Check sheet for the modelled part. Datum: model origin and axes. Units: mm. Face numbers are marked on the shaded views. Give positions to 0.01 mm unless a question says otherwise; leave off trailing zeros. Order: outer loops, then holes, each group sorted by start corner. A loop starts at its lowest first (then second) coordinate and runs counter-clockwise, first axis right, second up.
Item 1: Release check for a two-part mould opening along Z. For the marked faces 1, 2, 3 and 4 record: released by +Z, released by -Z, zero draft, split by the parting line, or undercut.
Item 2: Sectioned sample at A-A on y = 8. Record the boundary of the cut face in (x, z) (3 decimals).
Item 3: Sectioned sample at B-B on y = 3.5. Record the boundary of the cut face in (x, z) (3 decimals).
Item 4: Material ranges on line 1 along Y through (x, z) = (-0.25, 2.5); line 2 along Z through (x, y) = (1.25, 10.5) (3 decimals); line 3 along Y through (x, z) = (1, -0.75), recorded low to high.
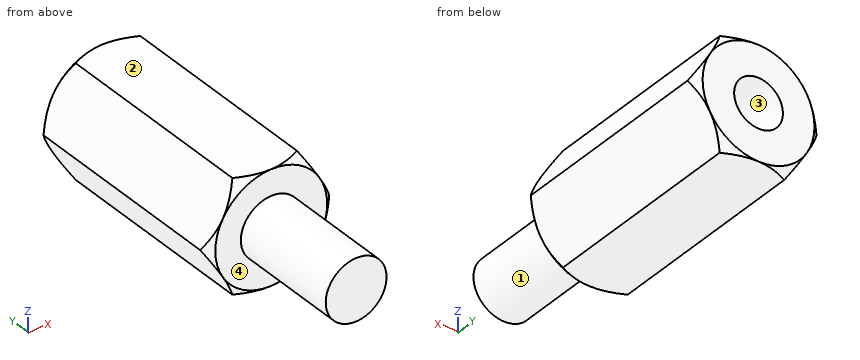
from build123d import *

# Parameters (mm, degrees)
BOSS_EXTRUDE1_DEPTH = 12.7
SKETCH5_R           = 1.3843
CUT_EXTRUDE1_DEPTH  = 6.35
SKETCH6_R           = 1.7272
BOSS_EXTRUDE2_DEPTH = 6.35


with BuildPart() as part:
    # Sketch1 → Boss-Extrude1 (new body)
    with BuildSketch(Plane(origin=(0, 0, 0), x_dir=(1, 0, 0), z_dir=(0, 1, 0))):
        Polygon((3.666174209, 0), (1.833087105, 3.175), (-1.833087105, 3.175), (-3.666174209, 0), (-1.833087105, -3.175), (1.833087105, -3.175), align=None)
    extrude(amount=BOSS_EXTRUDE1_DEPTH)

    # Sketch2 → Cut-Revolve1 (revolve, cut)
    with BuildSketch(Plane.XY):
        Polygon((-3.666174209, 0.491174209), (-3.175, 0), (-3.666174209, 0), align=None)
        Polygon((-3.666174209, 12.7), (-3.666174209, 12.208825791), (-3.175, 12.7), align=None)
    revolve(axis=Axis((0, 0, 0), (0, 1, 0)), mode=Mode.SUBTRACT)

    # Sketch5 → Cut-Extrude1 (cut)
    with BuildSketch(Plane(origin=(0, 12.7, 0), x_dir=(1, 0, 0), z_dir=(0, 1, 0))):
        with Locations(Location((0, 0, 0), (0, 0, 270))):
            Circle(SKETCH5_R)
    extrude(amount=-CUT_EXTRUDE1_DEPTH, mode=Mode.SUBTRACT)

    # Sketch6 → Boss-Extrude2 (add)
    with BuildSketch(Plane.XZ):
        with Locations(Location((0, 0, 0), (0, 0, 90))):
            Circle(SKETCH6_R)
    extrude(amount=BOSS_EXTRUDE2_DEPTH)


solid = part.part
Report:
1. face 1: split by the parting line
1. face 2: released by +Z
1. face 3: undercut
1. face 4: zero draft
2. outline: (-3.666, 0) - (-1.833, -3.175) - (1.833, -3.175) - (3.666, 0) - (1.833, 3.175) - (-1.833, 3.175) - close; hole circle Ø2.769 at (0, 0)
3. outline: (-3.666, 0) - (-1.833, -3.175) - (1.833, -3.175) - (3.666, 0) - (1.833, 3.175) - (-1.833, 3.175) - close
4. line 1: y = 0 to 12.7
4. line 2: z = -3.175 to -0.595, 0.595 to 3.175
4. line 3: y = -6.35 to 6.35
